Part model, mm, in its own coordinate system. A direction names the side the tool comes from. Coordinates: 2 decimals unless noted, no trailing zeros. Write each loop counter-clockwise with the first axis right and the second up, starting at its lowest first coordinate (ties: lowest second). Pieces come first, ordered by that corner, then holes. Notation, with made-up numbers: M 30,-10 L 49,-10 A24 ccw 49,17 Z; hole C -35,33 d7. An arc over 180 degrees is marked long. Use a Markdown table: item, result. Add a question column.
Q1. Tool access for faces 1 (the cylindrical face through (-4.437, -0.019, 2.465)), 2 (the cylindrical face through (-14.82, 12.94, 2.46)), 3 (the flat face through (-10, 8, 4)), 4 (the cylindrical face through (-21.966, -3.355, 3.655)): list every direction of +Z, -Z, +X, -X, +Y, -Y with a clear straight run to the whole face (end or side of a thin tool).
Q2. Slice it at B-B on z = 2.65. Write the cut outline in (x, y).
Q3. Wall check: L1, parallel to Y at x = -21.15, z = 2.5; L2, parallel to X at y = 4, z = 1.45; L3, parallel to Y at x = -17, z = 0.7. Give the ranges that are in metal, low to high. Write a range as from..to.
Q4. Mould opens along X. For faces 5 (the flat face through (-3, -8.376, 2)), 6 (the flat face through (-23.938, 2, 2)), 7 (the cylindrical face through (10.825, 9.864, 2.465)) say: released by +X, released by -X, zero draft, split by the parting line, or undercut.
Q5. Pin check, flat tips, straight feed: pin 1 Ø3 at (x, y) = (-9, 6.5) entering from -Z; pin 2 Ø1 at (x, y) = (16.06, 9.12) entering from +Z; pin 3 Ø1.5 at (x, z) = (-22, 3) entering from +Y; pin 4 Ø0.8 at (y, z) = (9.5, 3) entering from -X. Stop position of each tip, or through.
Q6. Slice it at A-A on x = 13.5. Write the cut outline in (y, z), then the cut area to 3 significant figures.
Q7. Slice it at C-C on y = -5. Write the cut outline in (x, z).
from build123d import *

# Parameters (mm, degrees)
SKETCH1_R           = 0.8
SKETCH1_R_2         = 3.5
SKETCH1_R_3         = 5.1
BOSS_EXTRUDE1_DEPTH = 5
SKETCH2_R           = 1.25
CUT_EXTRUDE1_DEPTH  = 4
BOSS_EXTRUDE2_START = -1
SKETCH21_R          = 5.1
BOSS_EXTRUDE2_DEPTH = 1


with BuildPart() as part:
    # Sketch1 → Boss-Extrude1 (new body)
    with BuildSketch(Plane(origin=(0, 0, 0), x_dir=(0, 1, 0), z_dir=(0, 0, 1))):
        with BuildLine():
            ThreePointArc((7.923715338, -23.061842121), (11.348253353, -21.704991773), (12.914157128, -18.370857874))
            Line((12.914157128, -18.370857874), (14.611258571, 9.036437401))
            ThreePointArc((14.611258571, 9.036437401), (14.470096631, 10.842810788), (13.835805455, 12.540039768))
            ThreePointArc((13.835805455, 12.540039768), (12.931450551, 14.850335933), (12.623684243, 17.312165753))
            Line((12.623684243, 17.312165753), (12.623684243, 23.938157879))
            Line((12.623684243, 23.938157879), (-8.376315757, 23.938157879))
            Line((-8.376315757, 23.938157879), (-8.376315757, -18.061842121))
            ThreePointArc((-8.376315757, -18.061842121), (-6.911849663, -21.597376027), (-3.376315757, -23.061842121))
            Line((-3.376315757, -23.061842121), (7.923715338, -23.061842121))
        make_face()
        with BuildLine():
            Line((-6.37591859, -2.133696229), (-6.376315757, -2.061842121))
            ThreePointArc((-6.376315757, -2.061842121), (0.123684243, 4.438157879), (6.623684243, -2.061842121))
            Line((6.623684243, -2.061842121), (6.623684243, -15.061842121))
            ThreePointArc((6.623684243, -15.061842121), (0.625179068, -21.542467318), (-6.298932046, -16.061842121))
            ThreePointArc((-6.298932046, -16.061842121), (-6.376216465, -15.097769724), (-6.309594086, -14.132901895))
            Line((-6.309594086, -14.132901895), (-6.37591859, -2.133696229))
        make_face(mode=Mode.SUBTRACT)
        with Locations(Location((9.123684243, -16.061842121, 0), (0, 0, 270))):
            Circle(SKETCH1_R, mode=Mode.SUBTRACT)
        with Locations(Location((9.623684243, -10.061842121, 0), (0, 0, 270))):
            Circle(SKETCH1_R, mode=Mode.SUBTRACT)
        with Locations(Location((9.123684243, -4.061842121, 0), (0, 0, 270))):
            Circle(SKETCH1_R, mode=Mode.SUBTRACT)
        with Locations(Location((1.537022692, 17.094912388, 0), (0, 0, 270))):
            Circle(SKETCH1_R_2, mode=Mode.SUBTRACT)
        with Locations(Location((8.123684243, 9.438157879, 0), (0, 0, 270))):
            Circle(SKETCH1_R_3, mode=Mode.SUBTRACT)
        with Locations(Location((5.623684243, 21.438157879, 0), (0, 0, 270))):
            Circle(SKETCH1_R, mode=Mode.SUBTRACT)
    extrude(amount=BOSS_EXTRUDE1_DEPTH)

    # Sketch2 → Cut-Extrude1 (cut)
    with BuildSketch(Plane(origin=(-23.938157879, 0, 0), x_dir=(0, -1, 0), z_dir=(-1, 0, 0))):
        with Locations(Location((-9.623684243, 2.5, 0), (0, 0, 90))):
            Circle(SKETCH2_R)
        with Locations(Location((2.876315757, 2.5, 0), (0, 0, 90))):
            Circle(SKETCH2_R)
    extrude(amount=-CUT_EXTRUDE1_DEPTH, mode=Mode.SUBTRACT)

    # Sketch21 → Boss-Extrude2 (add)
    with BuildSketch(Plane.XY.offset(5).offset(BOSS_EXTRUDE2_START)):
        with Locations((-9.438157879, 8.123684243)):
            Circle(SKETCH21_R)
    extrude(amount=BOSS_EXTRUDE2_DEPTH)


solid = part.part
Recorded:
| question | item | result |
|---|---|---|
| 1 | face 1 | +Z, -Z |
| 1 | face 2 | +Z, -Z, -X, +Y |
| 1 | face 3 | -Z |
| 1 | face 4 | -X |
| 2 | outline | M -23.94,-8.38 L 18.06,-8.38 A5 ccw 23.06,-3.38 L 23.06,7.92 A5 ccw 18.37,12.91 L -9.04,14.61 A6.5 ccw -12.54,13.84 A10 cw -17.31,12.62 L -23.94,12.62 L -23.94,10.86 L -19.94,10.86 L -19.94,8.38 L -23.94,8.38 L -23.94,-1.64 L -19.94,-1.64 L -19.94,-4.12 L -23.94,-4.12 Z; hole C -21.44,5.62 d1.6; hole C -17.09,1.54 d7; hole C -9.44,8.12 d10.2; hole M 2.06,-6.38 L 14.13,-6.31 A6.5 ccw long 15.06,6.62 L 2.06,6.62 A6.5 ccw Z; hole C 4.06,9.12 d1.6; hole C 10.06,9.62 d1.6; hole C 16.06,9.12 d1.6 |
| 3 | L1 | -8.38..-4.13, -1.63..4.88, 6.37..8.37, 10.87..12.62 |
| 3 | L2 | -23.94..-19.58, -14.61..-12.44, -6.44..-3.16, 20.28..23.06 |
| 3 | L3 | -8.38..-1.96, 5.04..12.63 |
| 4 | face 5 | zero draft |
| 4 | face 6 | released by -X |
| 4 | face 7 | undercut |
| 5 | pin 1 | z = 4 |
| 5 | pin 2 | through |
| 5 | pin 3 | y = 12.62 |
| 5 | pin 4 | x = -19.94 |
| 6 | outline | M -8.38,0 L -6.31,0 L -6.31,5 L -8.38,5 Z; M 6.62,0 L 13.22,0 L 13.22,5 L 6.62,5 Z |
| 6 | area | 43.3 mm² |
| 7 | outline | M -23.94,0 L -1.94,0 L -1.94,5 L -23.94,5 Z; M 19.06,0 L 22.79,0 L 22.79,5 L 19.06,5 Z |
